Design review of the part built by this model. Coordinates are the model's own, in mm. Face numbers are marked on the shaded views. A direction names the side the tool comes from. Coordinates: 2 decimals unless noted, no trailing zeros. Loops run counter-clockwise (first coordinate to the right, second up) from the corner with the lowest first, then second, coordinate; pieces in that order, holes last. Notation, with made-up numbers: (-29, 12.5) - (0, 12.5) arc R32 cw to (0, 49.5) - close; hole circle Ø11 at (31, 82). An arc over 180 degrees is marked (long way). One line per question, with ' | ' between items.
from build123d import *

# Parameters (mm, degrees)
PAD_DEPTH            = 30
PAD001_DEPTH         = 3.5
SKETCH002_W          = 13
SKETCH002_H          = 5
POCKET_DEPTH         = 33.501
SKETCH003_W          = 17.5
SKETCH003_H          = 9.5
POCKET001_DEPTH      = 30.5
POCKET002_DEPTH      = 120.501
POCKET002_DEPTH_BACK = -9.501
SKETCH008_W          = 9.5
SKETCH008_H          = 18
SKETCH008_H_2        = 11.637311
PAD002_DEPTH         = 1.6
SKETCH009_R          = 1.75
SKETCH009_R_2        = 1.5
POCKET003_DEPTH      = 22.001
POCKET003_DEPTH_BACK = -2.001


with BuildPart() as part:
    # Sketch → Pad (new body)
    with BuildSketch(Plane.XZ):
        Polygon((-55.5, 22), (-8.5, 22), (-8.5, 2), (8.5, 2), (8.5, 22), (55.5, 22), (55.5, 2), (65, 2), (65, 0), (55.5, 0), (55.5, -2), (8.5, -2), (8.5, 0), (-8.5, 0), (-8.5, -2), (-55.5, -2), (-55.5, 0), (-65, 0), (-65, 2), (-55.5, 2), align=None)
    extrude(amount=PAD_DEPTH)

    # Sketch001 → Pad001 (new body)
    with BuildSketch(Plane.XZ.offset(30)):
        with BuildLine():
            ThreePointArc((-52.5, 22), (-54.62132, 21.12132), (-55.5, 19))
            Line((-55.5, 19), (-55.5, 2))
            ThreePointArc((-55.5, 2), (-54.328434, -0.828421), (-51.500018, -2))
            Line((-51.500018, -2), (-12.499975, -2))
            ThreePointArc((-12.499975, -2), (-9.671566, -0.82842), (-8.5, 1.999996))
            Line((-8.5, 19.000001), (-8.5, 1.999996))
            ThreePointArc((-8.5, 19.000001), (-9.37868, 21.121321), (-11.5, 22))
            Line((-52.5, 22), (-11.5, 22))
        make_face()
        with BuildLine():
            ThreePointArc((11.5, 22), (9.37868, 21.12132), (8.5, 19))
            Line((8.5, 2), (8.5, 19))
            ThreePointArc((8.5, 2), (9.671573, -0.828427), (12.5, -2))
            Line((51.5, -2), (12.5, -2))
            ThreePointArc((51.5, -2), (54.328427, -0.828427), (55.5, 2))
            Line((55.5, 18.999976), (55.5, 2))
            ThreePointArc((55.5, 18.999976), (54.621329, 21.121312), (52.5, 22))
            Line((11.5, 22), (52.5, 22))
        make_face()
    extrude(amount=PAD001_DEPTH)

    # Sketch002 → Pocket (cut, through all)
    with BuildSketch(Plane(origin=(0, 0, 0), x_dir=(1, 0, 0), z_dir=(0, 1, 0))):
        with Locations((-32, -10)):
            Rectangle(SKETCH002_W, SKETCH002_H)
        with Locations((32, -10)):
            Rectangle(SKETCH002_W, SKETCH002_H)
    extrude(amount=-POCKET_DEPTH, mode=Mode.SUBTRACT)

    # Sketch003 → Pocket001 (cut)
    with BuildSketch(Plane(origin=(0, 0, 0), x_dir=(1, 0, 0), z_dir=(0, 1, 0))):
        with Locations((-32, -10)):
            Rectangle(SKETCH003_W, SKETCH003_H)
        with Locations((32, -10)):
            Rectangle(SKETCH003_W, SKETCH003_H)
    extrude(amount=-POCKET001_DEPTH, mode=Mode.SUBTRACT)

    # Sketch007 → Pocket002 (cut, two sides)
    with BuildSketch(Plane(origin=(55.5, 0, 0), x_dir=(0, 0, 1), z_dir=(1, 0, 0))) as pocket002_sk:
        Polygon((-2, 33.5), (22.001, 33.5), (22.001, 32.5), align=None)
    extrude(amount=-POCKET002_DEPTH, mode=Mode.SUBTRACT)
    extrude(pocket002_sk.sketch, amount=-POCKET002_DEPTH_BACK, mode=Mode.SUBTRACT)

    # Sketch008 → Pad002 (new body)
    with BuildSketch(Plane(origin=(0, 0, 0), x_dir=(1, 0, 0), z_dir=(0, 0, -1))):
        with Locations((-60.25, 9.50335)):
            Rectangle(SKETCH008_W, SKETCH008_H)
        with Locations((60.25, 13.927338)):
            Rectangle(SKETCH008_W, SKETCH008_H_2)
    extrude(amount=PAD002_DEPTH)

    # Sketch009 → Pocket003 (cut, two sides)
    with BuildSketch(Plane(origin=(0, 0, 0), x_dir=(1, 0, 0), z_dir=(0, 0, -1))) as pocket003_sk:
        with Locations((0, 19)):
            Circle(SKETCH009_R)
        with Locations((-60.5, 23)):
            Circle(SKETCH009_R_2)
        with Locations((-60.5, 14)):
            Circle(SKETCH009_R_2)
        with Locations((60.5, 23)):
            Circle(SKETCH009_R_2)
        with Locations((60.5, 14)):
            Circle(SKETCH009_R_2)
        with Locations((-60.5, 5)):
            Circle(SKETCH009_R_2)
    extrude(amount=-POCKET003_DEPTH, mode=Mode.SUBTRACT)
    extrude(pocket003_sk.sketch, amount=-POCKET003_DEPTH_BACK, mode=Mode.SUBTRACT)


solid = part.part
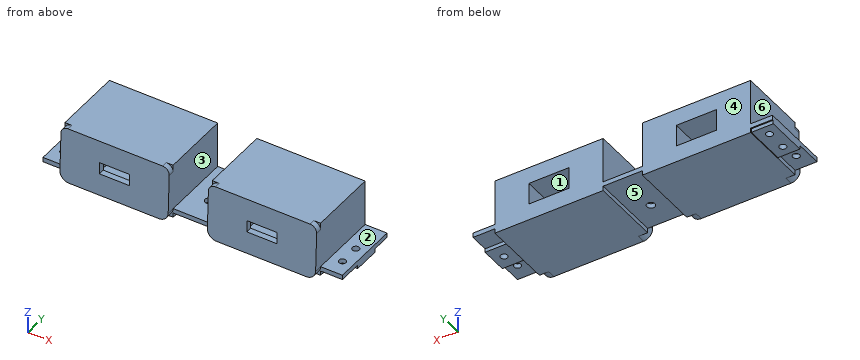
Q1. Tool access review of the marked faces 1, 2 and 3: name each direction out of +Z, -Z, +X, -X, +Y, -Y from which nothing blocks a thin tool from reaching the whole face with its end or side.
Returned:
face 1: +Y | face 2: +Z, +X, +Y, -Y | face 3: +Z, +Y, -Y
Q2. To check wall thickness, follow line 1 along X through (y, z) = (-22.5, 5.5); line 2 along X through (y, z) = (-23, 0.75); line 3 along Y through (x, z) = (-60.5, 0.1). State the ranges of each line that lie inside material, in increasing order.
Returned:
line 1: x = -55.5 to -40.75, -23.25 to -8.5, 8.5 to 23.25, 40.75 to 55.5 | line 2: x = -65 to -62, -59 to 59, 62 to 65 | line 3: y = -30 to -24.5, -21.5 to -15.5, -12.5 to -6.5, -3.5 to 0
Q3. Take a section at A-A (x = -60.5). Give the boundary of the cut face in (y, z).
Returned:
outline: (-30, 0) - (-24.5, 0) - (-24.5, 2) - (-30, 2) - close; (-21.5, 0) - (-18.5, 0) - (-18.5, -1.6) - (-15.5, -1.6) - (-15.5, 2) - (-21.5, 2) - close; (-12.5, -1.6) - (-6.5, -1.6) - (-6.5, 2) - (-12.5, 2) - close; (-3.5, -1.6) - (-0.5, -1.6) - (-0.5, 0) - (0, 0) - (0, 2) - (-3.5, 2) - close
Q4. Draft analysis for pull direction X (two halves, no side actions). For the marked faces 4, 5 and 6, state which applies: +X half, -X half, draft (parallel to the pull), parting line (faces both ways), or undercut.
Returned:
face 4: draft | face 5: undercut | face 6: -X half
Q5. For pin 1 (3.5 mm diameter, centred on x = -54.5, z = 21, fed in from -Y); pin 2 (5 mm diameter, centred on x = 3.5, y = -12.5, fed in from -Z); pin 3 (5 mm diameter, centred on x = -34, z = 7.5, fed in from +Y); pin 4 (10 mm diameter, centred on y = -19.5, z = 15, fed in from +X), all flat-tipped, find the tip position at first contact; note any pin that passes through.
Returned:
pin 1: stops at y = -32.61 | pin 2: stops at z = 0 | pin 3: stops at y = 0 | pin 4: stops at x = 55.5
Q6. Take a section at C-C (z = 17.5). Give the boundary of the cut face in (x, y), plus the area to 3 significant figures.
Returned:
outline: (-55.5, -32.69) - (-8.5, -32.69) - (-8.5, 0) - (-55.5, 0) - close; (8.5, -32.69) - (55.5, -32.69) - (55.5, 0) - (8.5, 0) - close | area: 3,070 mm²
Q7. Take a section at D-D (y = -23). State how many separate pieces and enclosed holes the cut face has, plus the area to 3 significant figures.
Returned:
separate pieces: 3 | enclosed holes: 2 | area: 1,980 mm²
Q8. Take a section at B-B (x = 36). Give the boundary of the cut face in (y, z).
Returned:
outline: (-33.5, -2) - (0, -2) - (0, 5.25) - (-30.5, 5.25) - (-30.5, 7.5) - (-33.1, 7.5) - close; (-32.9, 12.5) - (-30.5, 12.5) - (-30.5, 14.75) - (0, 14.75) - (0, 22) - (-32.5, 22) - close
